For this review, take the finished solid that the model builds, in its own axes (mm). Face numbers are marked on the shaded views. Round coordinates to 2 decimals unless told otherwise and drop trailing zeros. Write each loop counter-clockwise with the first axis right and the second up, starting at its lowest first coordinate (ties: lowest second). Pieces come first, ordered by that corner, then holes. Notation, with made-up numbers: M -31.5,-21.5 L -22.5,-21.5 A19 ccw -22.5,9.5 Z; hole C -36.5,-5.75 d4. An arc over 180 degrees is marked long. Answer in a Markdown table with one row per item.
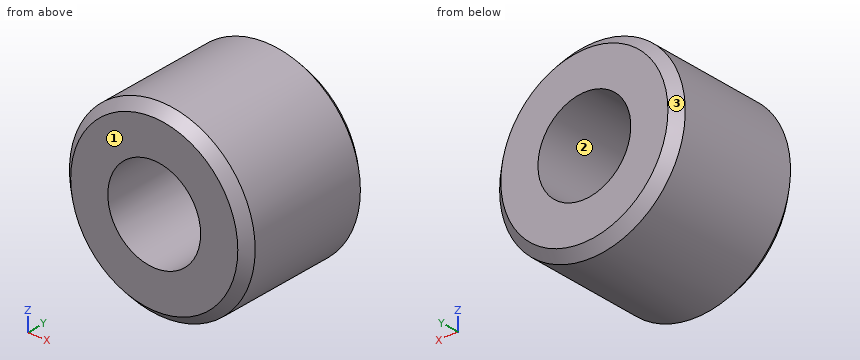
```python
from build123d import *

# Parameters (mm, degrees)
SKETCH1_R           = 10
BOSS_EXTRUDE1_DEPTH = 15
SKETCH2_R           = 5
CUT_EXTRUDE1_DEPTH  = 15
CHAMFER1_SIZE       = 1


with BuildPart() as part:
    # Sketch1 → Boss-Extrude1 (new body)
    with BuildSketch(Plane(origin=(0, 0, 0), x_dir=(1, 0, 0), z_dir=(0, 1, 0))):
        Circle(SKETCH1_R)
    extrude(amount=BOSS_EXTRUDE1_DEPTH)

    # Sketch2 → Cut-Extrude1 (cut)
    with BuildSketch(Plane(origin=(0, 15, 0), x_dir=(1, 0, 0), z_dir=(0, 1, 0))):
        Circle(SKETCH2_R)
    extrude(amount=-CUT_EXTRUDE1_DEPTH, mode=Mode.SUBTRACT)

    # Chamfer1
    chamfer1_edges = [part.edges().sort_by_distance(p)[0] for p in [
        (-10, 0, 0),
        (-10, 15, 0),
    ]]
    chamfer(chamfer1_edges, length=CHAMFER1_SIZE)


solid = part.part
```
Q1. For probe 1 along Z at (x, y) = (0, 3.5); probe 2 along X at (y, z) = (13.25, -2.25), list the stretches that pass through material, from the lowest coordinate up.
Found:
| item | result |
|---|---|
| probe 1 | -10 to -5, 5 to 10 |
| probe 2 | -9.74 to -4.47, 4.47 to 9.74 |
Q2. Take a section at B-B (z = 0). State the section outline as (x, y) points.
Found:
| item | result |
|---|---|
| outline | M -10,1 L -9,0 L -5,0 L -5,15 L -9,15 L -10,14 Z; M 5,0 L 9,0 L 10,1 L 10,14 L 9,15 L 5,15 Z |
Q3. Take a section at A-A (x = 0). State the section outline as (y, z) points.
Found:
| item | result |
|---|---|
| outline | M 0,-9 L 1,-10 L 14,-10 L 15,-9 L 15,-5 L 0,-5 Z; M 0,5 L 15,5 L 15,9 L 14,10 L 1,10 L 0,9 Z |
Q4. Take a section at C-C (y = 2.25). State the section outline as (x, z) points, then the cut area to 3 significant figures.
Found:
| item | result |
|---|---|
| outline | C 0,0 d20; hole C 0,0 d10 |
| area | 236 mm² |
Q5. Mouldability with a two-part tool opening along Z and no side actions: class the marked faces 1, 2 and 3 as +Z half, -Z half, draft (parallel to the pull), parting line (faces both ways), or undercut.
Found:
| item | result |
|---|---|
| face 1 | draft |
| face 2 | undercut |
| face 3 | parting line |
Q6. Insertion check: P1, Ø8, axis at x = 0, z = 0, coming from the +Y side; P2, Ø1, axis at x = -7.5, y = 12.5, coming from the +Z side; P3, Ø8, axis at y = 7, z = -6, coming from the +X side; P4, Ø2, axis at x = 7.5, z = -8, coming from the -Y side. Each pin has a flat end and moves straight along its axis. Give the tip position at first contact, or say it passes through.
Found:
| item | result |
|---|---|
| P1 | through |
| P2 | z = 7.14 |
| P3 | x = 9.8 |
| P4 | y = 0.97 |
